The figure shows three views and two pictorial views of one solid part (mm, origin at its lowest corner). Answer the questions. A direction names the side the tool comes from. Coordinates: 2 decimals unless noted, no trailing zeros. Loops run counter-clockwise (first coordinate to the right, second up) from the corner with the lowest first, then second, coordinate; pieces in that order, holes last. Notation, with made-up numbers: M 45,-4.5 L 60,-4.5 A27 cw 60,21.5 Z; hole C -23.75,36 d3. An arc over 180 degrees is marked long. Return JSON: item names as keys, results as strings. Group by question number.
1. Straight lines are drawn through the part: L1, parallel to Z at x = 10, y = 7.25 (3 decimals); L2, parallel to Z at x = 120.65, y = 8.75 (3 decimals); L3, parallel to X at y = 13.25, z = 76.2 (3 decimals). For each, find the intervals that lie inside material, in ascending order. Write a range as from..to.
2. Which of the six approach directions +Z, -Z, +X, -X, +Y, -Y give full straight-line access (tool end or side, diameter ignored) to the marked faces 4, 5 and 6?
3. Section C-C (y = 17.25) is taken. Count the separate pieces of the cut face and the enclosed holes in it, then the cut area to 3 significant figures.
4. Section B-B (z = 95) is taken. Write down the section's boundary in (x, y), then the cut area to 3 significant figures.
5. Section D-D (x = 14.5) is taken. Write down the section's boundary in (y, z).
6. The mould has two halves that part along Z. Classify the marked faces 1, 2 and 3: pulls with the +Z half, pulls with the -Z half, needs draft (parallel to the pull), parting line crosses it, or undercut.
7. Section A-A (x = 92) is taken. Write down the section's boundary in (y, z).
8. Given P1, Ø5.5, axis at x = 6.35, z = 123.825, coming from the -Y side; P2, Ø3, axis at x = 116.5, y = 15.5, coming from the -Z side (3 decimals); P3, Ø7.5, axis at y = 17, z = 134.5, coming from the -X side; P4, Ø7, axis at x = 11, y = 17.5, coming from the +Z side, each flat-ended and moving along its own axis, determine where each tip first touches the part or whether it passes through.
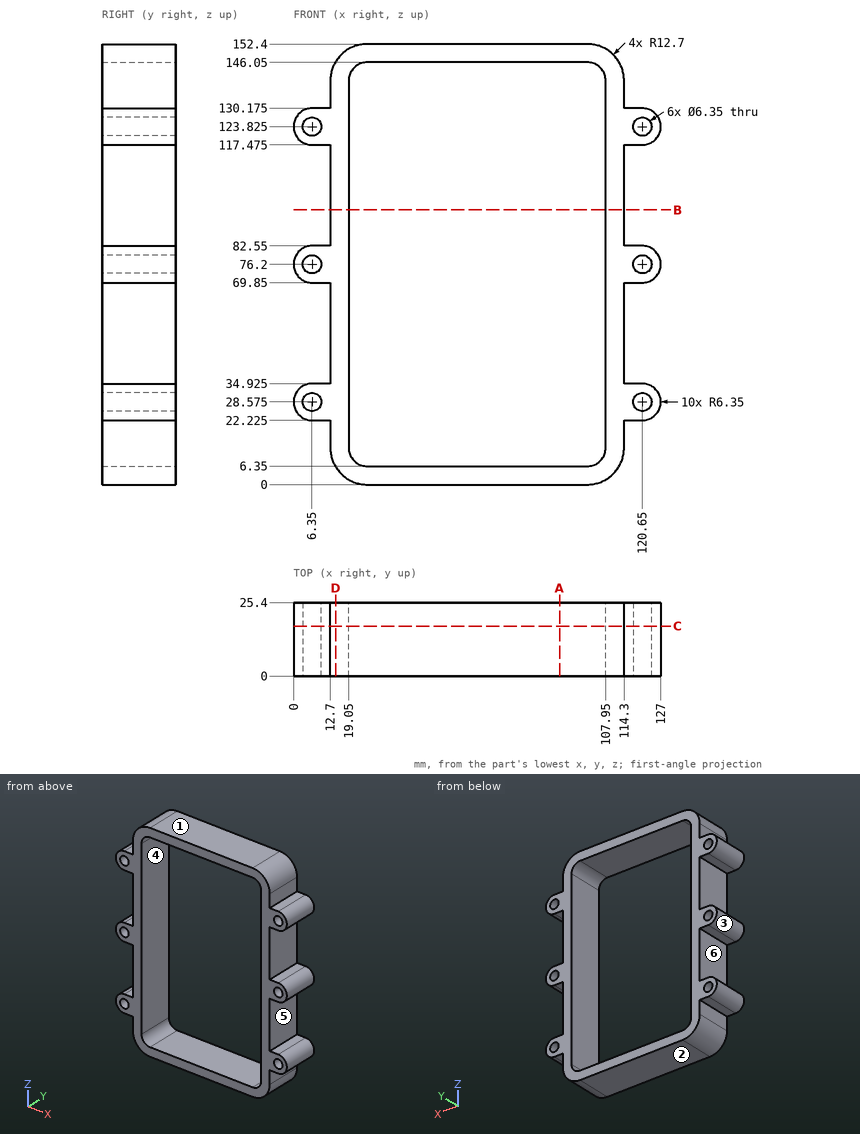
Worked out:
{
 "1": {"L1": "22.225..34.925, 69.85..82.55, 117.475..130.175", "L2": "22.225..25.4, 31.75..34.925, 69.85..73.025, 79.375..82.55, 117.475..120.65, 127..130.175", "L3": "0..3.175, 9.525..19.05, 107.95..117.475, 123.825..127"},
 "2": {"face 4": "+Y, -Y", "face 5": "+X, +Y, -Y", "face 6": "-X, +Y, -Y"},
 "3": {"separate pieces": "1", "enclosed holes": "7", "area": "3,630 mm^2"},
 "4": {"outline": "M 12.7,0 L 19.05,0 L 19.05,25.4 L 12.7,25.4 Z; M 107.95,0 L 114.3,0 L 114.3,25.4 L 107.95,25.4 Z", "area": "323 mm^2"},
 "5": {"outline": "M 0,6.18 L 25.4,6.18 L 25.4,146.22 L 0,146.22 Z"},
 "6": {"face 1": "pulls with the +Z half", "face 2": "pulls with the -Z half", "face 3": "undercut"},
 "7": {"outline": "M 0,0 L 25.4,0 L 25.4,6.35 L 0,6.35 Z; M 0,146.05 L 25.4,146.05 L 25.4,152.4 L 0,152.4 Z"},
 "8": {"P1": "through", "P2": "z = 22.225", "P3": "x = 12.7", "P4": "z = 146.22"}
}
